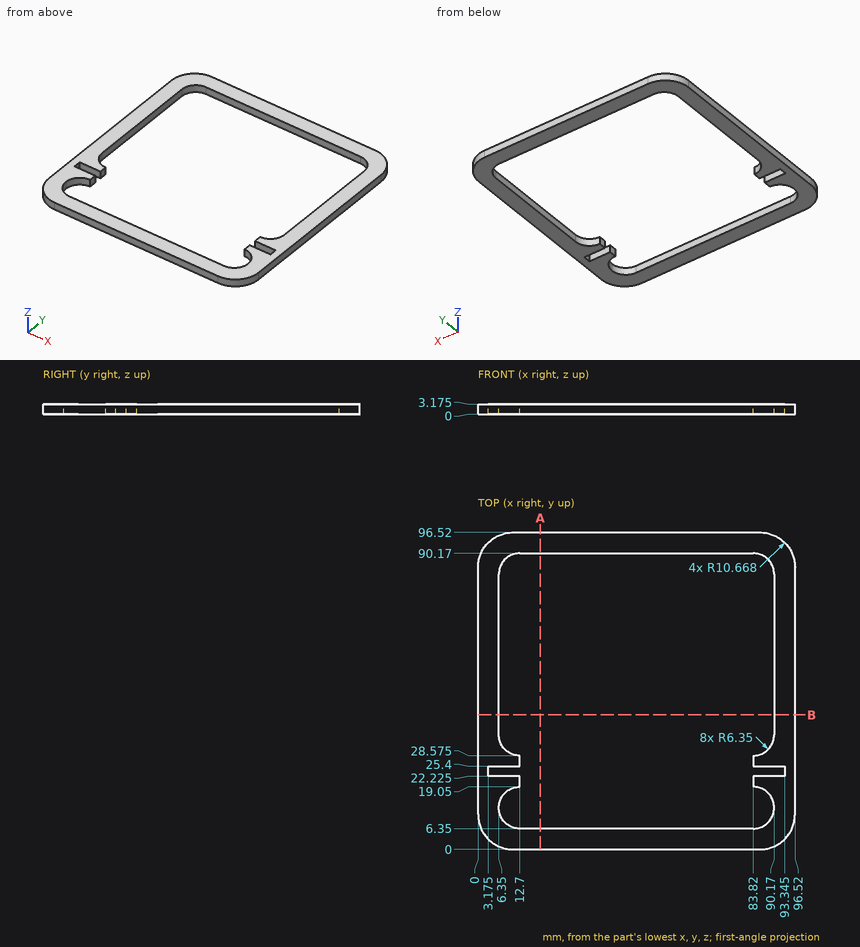
Check sheet for the drawn part. Datum: minimum x, y, z corner. Units: mm. Round coordinates to 2 decimals unless told otherwise and drop trailing zeros. Loops run counter-clockwise (first coordinate to the right, second up) from the corner with the lowest first, then second, coordinate; pieces in that order, holes last.
Item 1: Cross-section at A-A on x = 19. Record the boundary of the cut face in (y, z) (3 decimals), then the cut area to 3 significant figures.
Item 2: Gauge pin test, flat ends, axial feed: pin 1 (12 mm diameter, centred on x = 21.5, y = 36, fed in from +Z); pin 2 (1 mm diameter, centred on x = 88.5, z = 1, fed in from -Y); pin 3 (1.6 mm diameter, centred on x = 89.5, z = 1, fed in from +Y). Record the tip position at first contact, or that the pin passes through.
Item 3: Thickness scan on line 1 (Y direction, x = 65.5, z = 2.6); line 2 (X direction, y = 27, z = 2.3). Record the ranges inside material, lowest first.
Answer sheet:
1. outline: (0, 0) - (6.35, 0) - (6.35, 3.175) - (0, 3.175) - close; (90.17, 0) - (96.52, 0) - (96.52, 3.175) - (90.17, 3.175) - close
1. area: 40.3 mm2
2. pin 1: passes through
2. pin 2: stops at y = 0.22
2. pin 3: stops at y = 96.13
3. line 1: y = 0 to 6.35, 90.17 to 96.52
3. line 2: x = 0 to 12.7, 83.82 to 96.52
